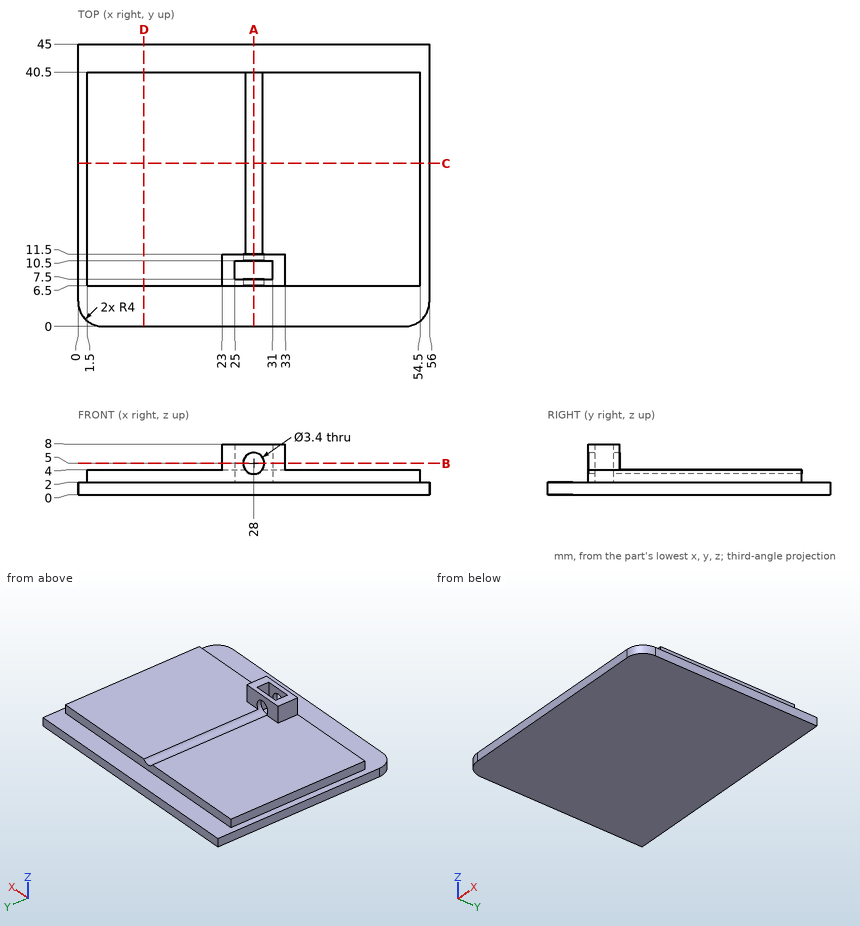
Study the drawing (mm; zero at the part's minimum x, y, z) and answer. Round coordinates to 2 decimals unless told otherwise and drop trailing zeros. Order: outer loops, then holes, each group sorted by start corner. A loop starts at its lowest first (then second) coordinate and runs counter-clockwise, first axis right, second up. Notation, with made-up numbers: (49.25, -24) -> (108.25, -24) arc R19 cw to (108.25, -2) -> close; hole circle Ø1 at (72, 12.25). An arc over 180 degrees is marked (long way). Answer as CSV lines item,"result". Start each with the question number.
(1) Find the intervals of material crossed by probe 1 along Y at (x, z) = (28, 2.5); probe 2 along Z at (x, y) = (3, 2); probe 3 along Z at (x, y) = (48, 13.5), in increasing order. Write a range as from..to.
(2) The part is cut by section C-C (y = 26). Determine the outline of the cut face in (x, z), then the cut area to 3 significant figures.
(3) The part is cut by section A-A (x = 28). Determine the outline of the cut face in (y, z), then the cut area to 3 significant figures.
(4) Flat-ended cylindrical pins translate along their axes: pin 1 Ø2 at (x, y) = (6.5, 29) entering from +Z; pin 2 Ø1 at (y, z) = (22.5, 3) entering from -X; pin 3 Ø1.5 at (y, z) = (9.5, 5.5) entering from -X. Find the tip coordinate at first contact, or state that the pin passes through.
(5) The part is cut by section D-D (x = 10.5). Determine the outline of the cut face in (y, z).
(6) The part is cut by section B-B (z = 5). Determine the outline of the cut face in (x, y), then the cut area to 3 significant figures.
Evaluation:
1,probe 1,"6.5..7.5, 10.5..40.5"
1,probe 2,"0..2"
1,probe 3,"0..4"
2,outline,"(0, 0) -> (56, 0) -> (56, 2) -> (54.5, 2) -> (54.5, 4) -> (29.37, 4) arc R1.7 cw to (26.63, 4) -> (1.5, 4) -> (1.5, 2) -> (0, 2) -> close"
2,area,"217 mm²"
3,outline,"(0, 0) -> (45, 0) -> (45, 2) -> (40.5, 2) -> (40.5, 3.3) -> (10.5, 3.3) -> (10.5, 2) -> (7.5, 2) -> (7.5, 3.3) -> (6.5, 3.3) -> (6.5, 2) -> (0, 2) -> close; (6.5, 6.7) -> (7.5, 6.7) -> (7.5, 8) -> (6.5, 8) -> close; (10.5, 6.7) -> (11.5, 6.7) -> (11.5, 8) -> (10.5, 8) -> close"
3,area,"133 mm²"
4,pin 1,"z = 4"
4,pin 2,"x = 1.5"
4,pin 3,"x = 23"
5,outline,"(0, 0) -> (45, 0) -> (45, 2) -> (40.5, 2) -> (40.5, 4) -> (6.5, 4) -> (6.5, 2) -> (0, 2) -> close"
6,outline,"(23, 6.5) -> (26.3, 6.5) -> (26.3, 7.5) -> (25, 7.5) -> (25, 10.5) -> (26.3, 10.5) -> (26.3, 11.5) -> (23, 11.5) -> close; (29.7, 6.5) -> (33, 6.5) -> (33, 11.5) -> (29.7, 11.5) -> (29.7, 10.5) -> (31, 10.5) -> (31, 7.5) -> (29.7, 7.5) -> close"
6,area,"25.2 mm²"
